The listing builds one solid part. Answer for the finished solid, in the listing's coordinates (mm). Round coordinates to 2 decimals unless told otherwise and drop trailing zeros. Loops run counter-clockwise (first coordinate to the right, second up) from the corner with the lowest first, then second, coordinate; pieces in that order, holes last. Notation, with made-up numbers: (8, -1) -> (53, -1) arc R20 ccw to (53, 37) -> close; hole circle Ø8 at (-37.75, 26.25). An arc over 180 degrees is marked (long way). Use a Markdown table: item, result. Add a question column.
Q1. Given pin 1 Ø3.5 at (x, z) = (0, 10.25) entering from +Y, flat-ended and moving along its own axis, determine where the tip first touches the part or whether it passes through.
Q2. Section A-A on x = 0 is taken. Give the vertices of the cut face in (y, z), then the cut area to 3 significant figures.
Q3. Consider line 1 (X direction, y = 0.35, z = 10.25); line 2 (Z direction, x = 0, y = -0.2); line 3 (Z direction, x = 8.25, y = 0.9). Determine where each line is inside the solid, lowest interval first.
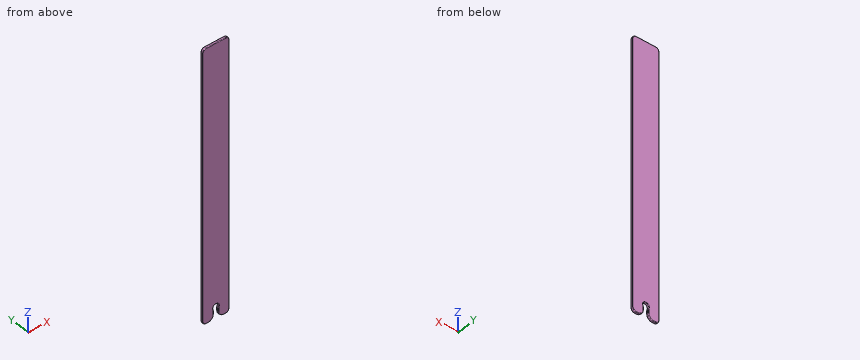
from build123d import *

# Parameters (mm, degrees)
F0_W          = 24
F0_H          = 2.2
F1_DEPTH      = 245
F3_DEPTH      = 1.101
F3_DEPTH_BACK = 1.101
F4_R          = 5
F5_R          = 3
F6_R          = 3
F7_R          = 0.5


with BuildPart() as f1:
    # F0 (on Top) → F1 (new body)
    with BuildSketch(Plane.XY):
        Rectangle(F0_W, F0_H)
    extrude(amount=F1_DEPTH)

    # F2 (on Front) → F3 (cut, two sides)
    with BuildSketch(Plane.XZ) as f3_sk:
        with BuildLine():
            Line((2.25, 0), (2.25, 8.6688611699))
            ThreePointArc((2.25, 8.6688611699), (0, 13), (-2.25, 8.6688611699))
            Line((-2.25, 8.6688611699), (-2.25, 0))
            Line((-2.25, 0), (2.25, 0))
        make_face()
    extrude(amount=-F3_DEPTH, mode=Mode.SUBTRACT)
    extrude(f3_sk.sketch, amount=F3_DEPTH_BACK, mode=Mode.SUBTRACT)

    # F4
    f4_edges = [f1.edges().sort_by_distance(p)[0] for p in [
        (2.25, 0, 0),
        (-2.25, 0, 0),
    ]]
    fillet(f4_edges, radius=F4_R)

    # F5
    f5_edges = [f1.edges().sort_by_distance(p)[0] for p in [
        (-2.25, 0, 8.668861),
        (2.25, 0, 8.668861),
    ]]
    fillet(f5_edges, radius=F5_R)

    # F6
    f6_edges = [f1.edges().sort_by_distance(p)[0] for p in [
        (12, 0, 245),
        (-12, 0, 245),
        (-12, 0, 0),
        (12, 0, 0),
    ]]
    fillet(f6_edges, radius=F6_R)

    # F7
    f7_edges = [f1.edges().sort_by_distance(p)[0] for p in [
        (-8.125, -1.1, 0),
        (-11.12132, -1.1, 0.87868),
        (-3.714466, -1.1, 1.464466),
        (-12, -1.1, 122.5),
        (-2.25, -1.1, 6.452396),
        (-11.12132, -1.1, 244.12132),
        (-2.315942, -1.1, 8.530335),
        (0, -1.1, 245),
        (0, -1.1, 13),
        (11.12132, -1.1, 244.12132),
        (2.315942, -1.1, 8.530335),
        (12, -1.1, 122.5),
        (2.25, -1.1, 6.452396),
        (11.12132, -1.1, 0.87868),
        (3.714466, -1.1, 1.464466),
        (8.125, -1.1, 0),
        (-8.125, 1.1, 0),
        (-11.12132, 1.1, 0.87868),
        (-3.714466, 1.1, 1.464466),
        (-12, 1.1, 122.5),
        (-2.25, 1.1, 6.452396),
        (-11.12132, 1.1, 244.12132),
        (-2.315942, 1.1, 8.530335),
        (0, 1.1, 245),
        (0, 1.1, 13),
        (11.12132, 1.1, 244.12132),
        (2.315942, 1.1, 8.530335),
        (12, 1.1, 122.5),
        (2.25, 1.1, 6.452396),
        (11.12132, 1.1, 0.87868),
        (3.714466, 1.1, 1.464466),
        (8.125, 1.1, 0),
    ]]
    fillet(f7_edges, radius=F7_R)


solid = f1.part
Checked values:
| question | item | result |
|---|---|---|
| 1 | pin 1 | passes through |
| 2 | outline | (-1.1, 13.5) arc R0.5 ccw to (-0.6, 13) -> (0.6, 13) arc R0.5 ccw to (1.1, 13.5) -> (1.1, 244.5) arc R0.5 ccw to (0.6, 245) -> (-0.6, 245) arc R0.5 ccw to (-1.1, 244.5) -> close |
| 2 | area | 510 mm2 |
| 3 | line 1 | x = -12 to -2.75, 2.75 to 12 |
| 3 | line 2 | z = 13 to 245 |
| 3 | line 3 | z = 0.1 to 244.9 |
